Check sheet for the modelled part. Datum: model origin and axes. Units: mm. Face numbers are marked on the shaded views. A direction names the side the tool comes from. Give positions to 0.01 mm unless a question says otherwise; leave off trailing zeros. Write each loop counter-clockwise with the first axis right and the second up, starting at its lowest first coordinate (ties: lowest second). Pieces come first, ordered by that corner, then holes. Notation, with made-up numbers: (37, 47) -> (55, 47) arc R27 cw to (55, 81) -> close; hole circle Ø1 at (9, 59.5). An arc over 180 degrees is marked (long way). Use a Markdown table: item, result. Add a question column.
1. Release check for a two-part mould opening along Y. For the marked faces 1, 2 and 3 record: released by +Y, released by -Y, zero draft, split by the parting line, or undercut.
2. Cross-section at C-C (x = 2.25). Enter the section's corners in (y, z).
3. Scan lines: probe 1 along Z at (x, y) = (4.5, 20); probe 2 along Z at (x, y) = (5.5, 4.5); probe 3 along Y at (x, z) = (7.25, 3.5). Record each from-to range of solid material in increasing order. Write a range as [from, to].
4. Gauge pin test, flat ends, axial feed: P1, Ø1.5, axis at x = 4, y = 1.5, coming from the -Z side; P2, Ø4, axis at y = 4, z = 2.5, coming from the +X side; P3, Ø3, axis at y = 20, z = 5, coming from the -X side; P4, Ø4, axis at x = 8.5, z = 9, coming from the +Y side. Record the tip position at first contact, or that the pin passes through.
5. Cross-section at D-D (y = 23.25). Enter the section's corners in (x, z), then the cut area to 3 significant figures.
6. Cross-section at B-B (z = 6.25). Enter the section's corners in (x, y), then the cut area to 3 significant figures.
7. Set-up check for the marked faces 4 and 5: record each of +Z, -Z, +X, -X, +Y, -Y from which the full face is reachable in a straight line by a thin tool's end or side.
8. Cross-section at A-A (y = 18.5). Enter the section's corners in (x, z).
from build123d import *

# Parameters (mm, degrees)
SKETCH_W     = 10
SKETCH_H     = 20
PAD_DEPTH    = 5
SKETCH001_W  = 10
SKETCH001_H  = 25
PAD001_DEPTH = 5
SKETCH002_R  = 2
POCKET_DEPTH = 10


with BuildPart() as part:
    # Sketch → Pad (new body)
    with BuildSketch(Plane.XY):
        with Locations((5, 15)):
            Rectangle(SKETCH_W, SKETCH_H)
    extrude(amount=PAD_DEPTH)

    # Sketch001 → Pad001 (new body)
    with BuildSketch(Plane.XY.offset(5)):
        with Locations((5, 12.5)):
            Rectangle(SKETCH001_W, SKETCH001_H)
    extrude(amount=PAD001_DEPTH)

    # Sketch002 → Pocket (cut)
    with BuildSketch(Plane.YZ.offset(10)):
        with Locations((20, 5)):
            Circle(SKETCH002_R)
        with BuildLine():
            ThreePointArc((25, 5), (23.535534, 8.535534), (20, 10))
            Line((20, 10), (25, 10))
            Line((25, 10), (25, 5))
        make_face()
        with BuildLine():
            ThreePointArc((20.00002, 0), (23.535546, 1.464468), (25, 5))
            Line((25, 0), (25, 5))
            Line((20.00002, 0), (25, 0))
        make_face()
    extrude(amount=-POCKET_DEPTH, mode=Mode.SUBTRACT)


solid = part.part
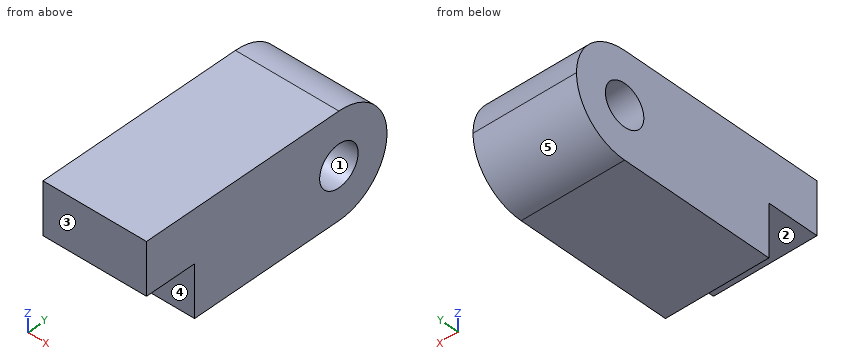
Worked answers:
| question | item | result |
|---|---|---|
| 1 | face 1 | undercut |
| 1 | face 2 | zero draft |
| 1 | face 3 | released by -Y |
| 2 | outline | (0, 5) -> (5, 5) -> (5, 0) -> (20, 0) arc R5 ccw to (25, 5) arc R5 ccw to (20, 10) -> (0, 10) -> close; hole circle Ø4 at (20, 5) |
| 3 | probe 1 | z = [0, 3], [7, 10] |
| 3 | probe 2 | z = [5, 10] |
| 3 | probe 3 | y = [5, 18.68], [21.32, 24.77] |
| 4 | P1 | stops at z = 5 |
| 4 | P2 | stops at x = 10 |
| 4 | P3 | passes through |
| 4 | P4 | stops at y = 24.58 |
| 5 | outline | (0, 1.2) -> (10, 1.2) -> (10, 8.8) -> (0, 8.8) -> close |
| 5 | area | 76.0 mm² |
| 6 | outline | (0, 0) -> (10, 0) -> (10, 18.44) -> (0, 18.44) -> close; (0, 21.56) -> (10, 21.56) -> (10, 24.84) -> (0, 24.84) -> close |
| 6 | area | 217 mm² |
| 7 | face 4 | -Z, +X, -X, -Y |
| 7 | face 5 | -Z, +X, -X, +Y |
| 8 | outline | (0, 0) -> (10, 0) -> (10, 3.68) -> (0, 3.68) -> close; (0, 6.32) -> (10, 6.32) -> (10, 10) -> (0, 10) -> close |
